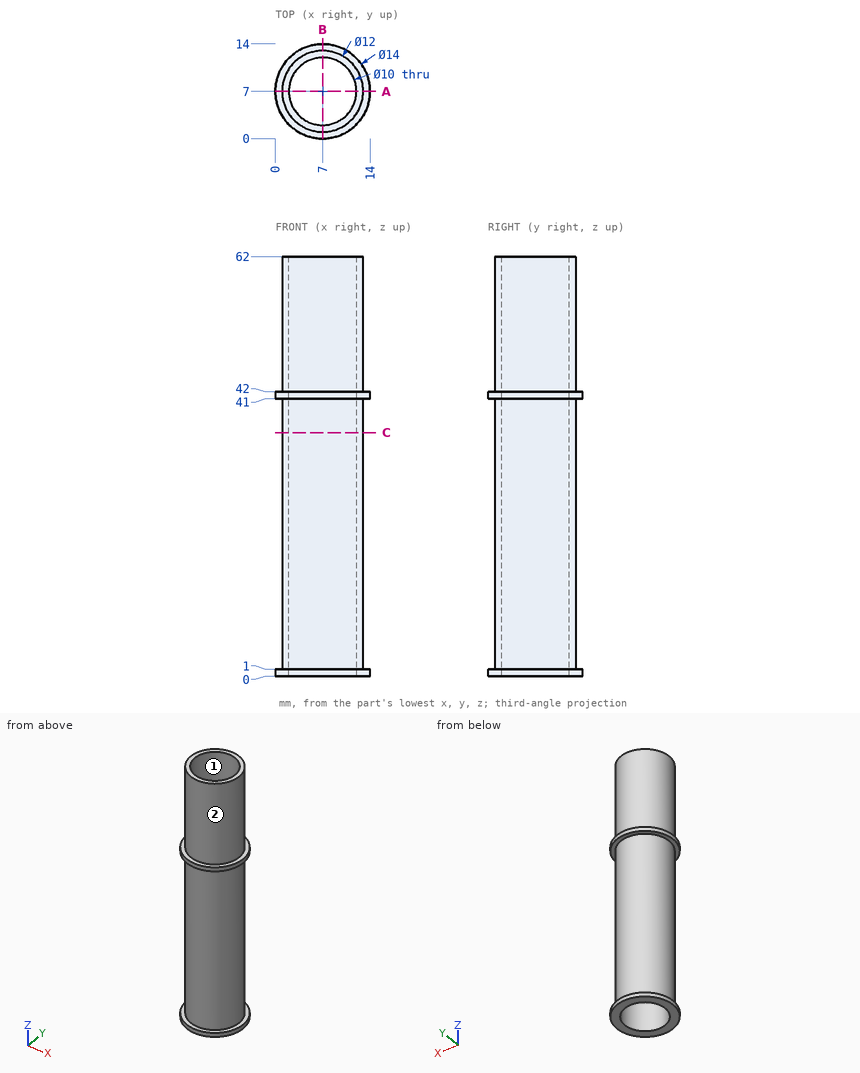
For this review, use the dimensioned drawing (mm, ordinates from the lowest corner) and the shaded views. Coordinates: 2 decimals unless noted, no trailing zeros. Order: outer loops, then holes, each group sorted by start corner. A loop starts at its lowest first (then second) coordinate and runs counter-clockwise, first axis right, second up. Notation, with made-up numbers: (-7, 49) - (36, 49) arc R11 cw to (36, 60) - close; hole circle Ø2 at (79, 72). An arc over 180 degrees is marked (long way). Answer in a Markdown table with one row per item.
(1) Wall thickness on line 1 along Y through (x, z) = (7, 18.5); line 2 along Y through (x, z) = (3.75, 54); line 3 along Z through (x, y) = (7.75, 1): over which ranges is each line inside the solid? List them lowest first. Write a range as from..to.
Checked values:
| item | result |
|---|---|
| line 1 | 1..2, 12..13 |
| line 2 | 1.96..3.2, 10.8..12.04 |
| line 3 | 0..1, 41..42 |
(2) Consider section A-A on y = 7. State the section outline as (x, z) points, plus the area to 3 significant figures.
Checked values:
| item | result |
|---|---|
| outline | (0, 0) - (2, 0) - (2, 62) - (1, 62) - (1, 42) - (0, 42) - (0, 41) - (1, 41) - (1, 1) - (0, 1) - close; (12, 0) - (14, 0) - (14, 1) - (13, 1) - (13, 41) - (14, 41) - (14, 42) - (13, 42) - (13, 62) - (12, 62) - close |
| area | 128 mm^2 |
(3) The part is to be moulded in two halves that separate along X. For the marked faces 1 and 2, say which applies: released by +X, released by -X, zero draft, split by the parting line, or undercut.
Checked values:
| item | result |
|---|---|
| face 1 | undercut |
| face 2 | split by the parting line |
(4) Clearance check with flat-ended pins moving along their axes: pin 1 (1 mm diameter, centred on x = 4.5, z = 8, fed in from +Y); pin 2 (3 mm diameter, centred on y = 12.5, z = 17, fed in from +X); pin 3 (5 mm diameter, centred on y = 5.5, z = 49, fed in from +X); pin 4 (6 mm diameter, centred on x = 7, y = 7, fed in from -Z). State where each tip first meets the part, or that it passes through.
Checked values:
| item | result |
|---|---|
| pin 1 | y = 12.66 |
| pin 2 | x = 11.47 |
| pin 3 | x = 13 |
| pin 4 | through |
(5) Consider section C-C on z = 36. State the section outline as (x, y) points.
Checked values:
| item | result |
|---|---|
| outline | circle Ø12 at (7, 7); hole circle Ø10 at (7, 7) |
